Verification items for the finished model (mm, model axes). A direction names the side the tool comes from. Coordinates: 2 decimals unless noted, no trailing zeros. Order: outer loops, then holes, each group sorted by start corner. A loop starts at its lowest first (then second) coordinate and runs counter-clockwise, first axis right, second up. Notation, with made-up numbers: M -7,16 L 51,16 A26 cw 51,34 Z; hole C -6.5,84 d11. An arc over 180 degrees is marked long. Return JSON: item names as keys, results as strings.
Autodesk Fusion 360 part; units mm, degrees
sketch "Sketch1" plane through (0, 0, 0) normal (0, 0, 1) x (1, 0, 0)
  line L0 (0, 0) -> (27.04, 0)
  line L1 (27.04, 0) -> (27.04, -1.2)
  line L2 (27.04, -1.2) -> (0, -1.2)
  line L3 (0, -1.2) -> (0, 0)
  dimension "d1" = 27.04
  dimension "d2" = 1.2
extrude "Extrude1" add sketch "Sketch1" along normal blind 4
sketch "Sketch2" plane through (0, -1.2, 0) normal (0, -1, 0) x (1, 0, 0)
  line L0 (0, 0) -> (27.04, 0)
  line L1 (27.04, 0) -> (27.04, 4)
  line L2 (27.04, 4) -> (0, 4)
  line L3 (0, 4) -> (0, 0)
  circle A0 centre (27.04, 2) radius 2
  dimension "d5" = 4
extrude "Extrude2" add sketch "Sketch2" against normal blind 1.2 contours L1 A0 picked at (27.2278, 2.6397)
sketch "Sketch3" plane through (0, -1.2, 0) normal (0, -1, 0) x (1, 0, 0)
  line L0 (0, 0) -> (27.04, 0)
  arc A0 (27.04, 0) -> (27.04, 4) centre (27.04, 2) ccw
  line L1 (27.04, 4) -> (0, 4)
  line L2 (0, 4) -> (0, 0)
  circle A1 centre (27.04, 2) radius 0.7
  dimension "d8" = 1.4
extrude "Extrude3" cut sketch "Sketch3" against normal blind 10 contours A1
sketch "Sketch4" plane through (0, -1.2, 0) normal (0, -1, 0) x (1, 0, 0)
  circle A0 centre (27.04, 2) radius 0.7
  line L0 (0, 0) -> (27.04, 0)
  arc A1 (27.04, 0) -> (27.04, 4) centre (27.04, 2) ccw
  line L1 (27.04, 4) -> (0, 4)
  line L2 (0, 4) -> (0, 0)
  line L3 (0, 0) -> (0, 1.5)
  circle A2 centre (0, 1.5) radius 1.5
  line L4 (-1.0715, 0) -> (5.393, 0) construction
  line L5 (-0.8097, 0) -> (6.2004, 0) construction
  line L6 (25.3, 0) -> (25.3, 4)
  line L7 (25.3, 0) -> (29.5592, 0)
  line L8 (25.3, 4) -> (30.5, 4)
  line L9 (29.04, 0) -> (29.04, 4)
  line L10 (29.04, 4) -> (1.69, 4)
  line L11 (29.04, 4) -> (1.69, 4)
  line L12 (29.04, 4) -> (1.69, 4)
  line L13 (1.69, 4) -> (-0.31, 4)
  circle A3 centre (-0.31, 4) radius 2
  line L14 (1.69, 4) -> (-2.28, 4)
  line L15 (-2.28, 4) -> (-2.28, 4.3451)
  line L16 (1.69, 4) -> (-2.28, 4.3451)
  line L17 (-0.7906, 0) -> (-2.7155, 5.6156)
  line L18 (-0.7906, 0) -> (6.1719, 0) construction
  line L19 (-2.28, 4) -> (29.04, 4)
  dimension "d11" = 1.5
  dimension "d12" = 3
  dimension "d23" = 27.35
  dimension "d24" = 180
  dimension "d25" = 27.35
  dimension "d26" = 2
  dimension "d27" = 4
  dimension "d28" = 3.97
  dimension "d29" = 108.92
  dimension "d30" = 31.32
extrude "Extrude4" add sketch "Sketch4" against normal blind 1.2 contours L2 L3 A2 A3 L17 | L2 L3 A2 A3 | A2 A3 L17 | A3 L16 | L1 L13 L14 L16 L17 L19 | L2 A2 L13 A3 L14 L17 L19
sketch "Sketch5" plane through (0, -1.2, 0) normal (0, -1, 0) x (1, 0, 0)
  circle A0 centre (27.04, 2) radius 0.7
  line L0 (0, 0) -> (27.04, 0)
  arc A1 (27.04, 0) -> (27.04, 4) centre (27.04, 2) ccw
  line L1 (27.04, 4) -> (1.69, 4)
  arc A2 (1.69, 4) -> (-2.28, 4.3451) centre (-0.31, 4) ccw
  line L2 (-2.28, 4.3451) -> (-0.8912, 0.2935)
  arc A3 (-0.8912, 0.2935) -> (0, 0) centre (0, 1.5) ccw
  circle A4 centre (27.04, 2) radius 0.7
  dimension "d37" = 1.4
sketch "Sketch6" plane through (0, -1.2, 0) normal (0, -1, 0) x (1, 0, 0)
  circle A0 centre (-0.3, 4) radius 0.7
  dimension "d34" = 1.4
extrude "Extrude5" cut sketch "Sketch6" against normal blind 6.5
sketch "Sketch7" plane through (0, -1.2, 0) normal (0, -1, 0) x (1, 0, 0)
extrude "Extrude6" add sketch "Sketch5" against normal blind 1.95 contours A0 A4
extrude "Extrude7" add 1 faces at (26.8677, 0.75, 1.935) along direction (0, -1, 0) blind 2.7
Q1. Draft check along Z on faces 1 (the face through (0, -0.6, 2.5)), 2 (the face through (14, -1, 4)), 3 (the face through (27, 0.75, 2)). Enter one of: pulls with the +Z half, pulls with the -Z half, needs draft (parallel to the pull), parting line crosses it, or undercut.
Values:
{"face 1": "undercut", "face 2": "pulls with the +Z half", "face 3": "needs draft"}
Q2. Cross-section at A-A, the plane y = -0.6. Record the boundary of the cut face in (x, z).
Values:
{"outline": "M -2.28,4.35 L -0.89,0.29 A1.5 ccw 0,0 L 27.04,0 A2 ccw 27.04,4 L 1.69,4 A2 ccw Z; hole M -1.29,2.26 A2 ccw 0,2.02 L 0,3 A1.5 ccw Z; hole C -0.3,4 d1.4"}
Q3. Material ranges on line 1 along Z through (x, y) = (-0.3, -0.8); line 2 along Y through (x, z) = (22, 2.5); line 3 along Z through (x, y) = (17, -0.65), recorded low to high.
Values:
{"line 1": "0.03 to 2, 2.97 to 3.3, 4.7 to 6", "line 2": "-1.2 to 0", "line 3": "0 to 4"}
Q4. Tool access check on faces 4 (the face through (-0.1, -0.61, 5.99)), 5 (the face through (26.34, 0.37, 2.03)), 6 (the face through (26.34, -1.57, 1.97)). Record the directions out of +Z, -Z, +X, -X, +Y, -Y that give a thin tool (end or side, any length) a straight path to the whole face; none if there is none.
Values:
{"face 4": "+Z, +Y, -Y", "face 5": "+Y", "face 6": "-Y"}
Q5. Cross-section at C-C, the plane x = -0.3. Record the boundary of the cut face in (y, z), and give its area (3 significant figures).
Values:
{"outline": "M -1.2,0.03 L 0,0.03 L 0,2 L -1.2,2 Z; M -1.2,2.97 L 0,2.97 L 0,3.3 L -1.2,3.3 Z; M -1.2,4.7 L 0,4.7 L 0,6 L -1.2,6 Z", "area": "4.32 mm^2"}
Q6. Go/stop test with flat-tipped pins: pin 1 (2 mm diameter, centred on x = -0.3, z = 4, fed in from -Y); pin 2 (0.5 mm diameter, centred on y = -1, z = 2.5, fed in from -X). Record where each tip stops, or that it passes through.
Values:
{"pin 1": "y = -1.2", "pin 2": "x = -1.73"}
Q7. Cross-section at D-D, the plane x = 19. Record the boundary of the cut face in (y, z).
Values:
{"outline": "M -1.2,0 L 0,0 L 0,4 L -1.2,4 Z"}
Q8. Cross-section at B-B, the plane z = 3.7. Record the boundary of the cut face in (x, y), and give its area (3 significant figures).
Values:
{"outline": "M -2.06,-1.2 L -0.93,-1.2 L -0.93,0 L -2.06,0 Z; M 0.33,-1.2 L 28.09,-1.2 L 28.09,0 L 0.33,0 Z", "area": "34.7 mm^2"}
